```python
from build123d import *

# Parameters (mm, degrees)
F1_DEPTH = 3
F3_DEPTH = 3


with BuildPart() as f1:
    # F0 (on Front) → F1 (new body)
    with BuildSketch(Plane.XZ):
        with BuildLine():
            Line((-26.2521904707, -26.5712421387), (26.2521904707, -26.5712421387))
            ThreePointArc((26.2521904707, -26.5712421387), (29.7877243766, -25.1067760447), (31.2521904707, -21.5712421387))
            Line((31.2521904707, -21.5712421387), (31.2521904707, 21.5712421387))
            ThreePointArc((31.2521904707, 21.5712421387), (29.7877243766, 25.1067760447), (26.2521904707, 26.5712421387))
            Line((26.2521904707, 26.5712421387), (-26.2521904707, 26.5712421387))
            ThreePointArc((-26.2521904707, 26.5712421387), (-29.7877243766, 25.1067760447), (-31.2521904707, 21.5712421387))
            Line((-31.2521904707, 21.5712421387), (-31.2521904707, -21.5712421387))
            ThreePointArc((-31.2521904707, -21.5712421387), (-29.7877243766, -25.1067760447), (-26.2521904707, -26.5712421387))
        make_face()
        with BuildLine():
            Line((-24.1804867983, 6.5188668668), (-24.1804867983, 19.0295055509))
            Line((-24.1804867983, 19.0295055509), (-9.5692276955, 19.0295055509))
            Line((-9.5692276955, 19.0295055509), (-9.5692276955, 14.7253833711))
            Line((-9.5692276955, 14.7253833711), (-18.7460067018, 14.7253833711))
            ThreePointArc((-18.7460067018, 14.7253833711), (-19.0189579715, 14.6123232533), (-19.1320180893, 14.3393719836))
            Line((-19.1320180893, 14.3393719836), (-19.1320180893, 11.5628045595))
            ThreePointArc((-19.1320180893, 11.5628045595), (-19.052543922, 11.4032002875), (-18.8772828528, 11.3704401816))
            add(Edge.make_bspline(
                [(-18.8772828528, 11.3704401816), (-18.0907039553, 11.5942528357), (-16.428571119, 12.048986212), (-13.7637590064, 12.1663926481), (-10.7783023467, 11.2878918717), (-8.608008816, 8.883739189), (-7.8235892044, 7.195407339), (-7.479812433, 6.4214548917)],
                knots=[0.0187889452, 0.0187889452, 0.0187889452, 0.0187889452, 0.1928215696, 0.3859968189, 0.5892635727, 0.8004585236, 0.9781550685, 0.9781550685, 0.9781550685, 0.9781550685], degree=3))
            ThreePointArc((-7.479812433, 6.4214548917), (-7.1773938737, 6.1954394373), (-6.8268028651, 6.3355319618))
            add(Edge.make_bspline(
                [(-6.8268028651, 6.3355319618), (-6.3239368021, 6.9578108483), (-5.1657820011, 8.33523566), (-2.1396728387, 9.9326729538), (1.8950429815, 10.0853631714), (6.0194775368, 7.6605840045), (8.3949703412, 3.199174132), (8.7962173797, 0.4841619269), (8.9867115021, -0.8048042655)],
                knots=[0.0134429235, 0.0134429235, 0.0134429235, 0.0134429235, 0.1392843233, 0.2952512735, 0.4619051388, 0.6427907875, 0.8304130649, 1, 1, 1, 1], degree=3))
            Line((8.9867115021, -0.8048042655), (12.9019767046, -0.2800785005))
            add(Edge.make_bspline(
                [(12.9019767046, -0.2800785005), (13.0543244929, -1.4128068863), (13.328107964, -3.4484279333), (14.1004293769, -5.4535206804), (15.2062121625, -6.7542628508), (17.2121585921, -7.2105429933), (19.0659013385, -6.2089714944), (19.9198257488, -4.6565826928), (20.2026522486, -0.8100851133), (20.0692985967, 3.029626915), (20.2545182868, 5.7747033617), (18.5907316712, 8.3373482447), (16.4047076085, 8.7783260416), (14.8198998378, 8.6742253566), (13.28172228, 7.3709317022), (13.085235865, 6.1267789414), (12.9698067904, 5.5243223906)],
                knots=[0, 0, 0, 0, 0.0850530681, 0.1531982013, 0.2128134932, 0.2778382163, 0.3433024412, 0.4040377865, 0.4960108059, 0.5899390151, 0.6674603836, 0.7458264942, 0.8140016254, 0.8723646786, 0.9361011897, 1, 1, 1, 1], degree=3))
            Line((12.9698067904, 5.5243223906), (8.4308534861, 6.5188668668))
            Line((8.4308534861, 6.5188668668), (8.4308534861, 19.0295055509))
            Line((8.4308534861, 19.0295055509), (23.0421125889, 19.0295055509))
            Line((23.0421125889, 19.0295055509), (23.0421125889, 14.7253833711))
            Line((23.0421125889, 14.7253833711), (13.8653335825, 14.7253833711))
            ThreePointArc((13.8653335825, 14.7253833711), (13.5923823128, 14.6123232533), (13.4793221951, 14.3393719836))
            Line((13.4793221951, 14.3393719836), (13.4793221951, 11.5626012477))
            ThreePointArc((13.4793221951, 11.5626012477), (13.5587386682, 11.40304056), (13.7339183255, 11.370197343))
            add(Edge.make_bspline(
                [(13.7339183255, 11.370197343), (14.5206329081, 11.5934338311), (16.1829432155, 12.0472832886), (18.8464510581, 12.1747073507), (21.8375982381, 11.2543430537), (24.2004389296, 8.7818679608), (25.5755735256, 4.8713271716), (25.3064350862, -0.5737911857), (24.8312041176, -4.7094018545), (21.749976272, -9.0376680335), (16.9706732988, -10.4786564529), (12.5389209811, -9.3007692118), (10.8350653675, -7.5140693006), (10.3080651221, -6.5522620029)],
                knots=[0.006673314, 0.006673314, 0.006673314, 0.006673314, 0.0685294658, 0.1371846306, 0.2094263518, 0.2844857821, 0.3685608886, 0.4653028232, 0.5506041076, 0.6431140813, 0.7339975358, 0.8229147331, 0.8907000755, 0.8907000755, 0.8907000755, 0.8907000755], degree=3))
            ThreePointArc((10.3080651221, -6.5522620029), (9.8768736928, -6.3630255441), (9.583580391, -6.731421425))
            add(Edge.make_bspline(
                [(-8.4416717291, -13.5454395786), (-7.9438695099, -14.71578707), (-6.9579408758, -17.0337339557), (-4.2409263056, -19.6699254166), (0.459261844, -20.936928095), (5.9462638445, -19.1007566385), (8.4575100908, -14.8113966737), (9.4779663102, -10.267236628), (9.5666941787, -7.7613995922), (9.583580391, -6.731421425)],
                knots=[0, 0, 0, 0, 0.131573279, 0.2605891623, 0.4072468832, 0.5651074981, 0.7133867816, 0.8642572868, 0.9719474004, 0.9719474004, 0.9719474004, 0.9719474004], degree=3))
            Line((-8.4416717291, -13.5454395786), (-3.91946733, -12.3001933098))
            add(Edge.make_bspline(
                [(3.4391110044, -8.801032884), (3.4292294296, -9.8788771881), (3.3907020801, -12.0466383407), (2.98547267, -14.7224859441), (1.1638632401, -16.8474068921), (-1.2378962082, -16.8165054966), (-3.15517022, -15.3270751162), (-3.6508764536, -13.3639063953), (-3.91946733, -12.3001933098)],
                knots=[0.0310308646, 0.0310308646, 0.0310308646, 0.0310308646, 0.1949538702, 0.364973689, 0.5249423704, 0.6722147355, 0.8223945444, 1, 1, 1, 1], degree=3))
            ThreePointArc((3.4391110044, -8.801032884), (3.2178473715, -8.4483976929), (2.804982612, -8.5018005366))
            add(Edge.make_bspline(
                [(-7.6247713503, -5.0285945502), (-7.4951246028, -5.4581028515), (-7.1182427223, -6.5417591982), (-5.5143339169, -8.3435497571), (-1.8620178866, -10.0886878273), (1.4142697444, -9.5568731886), (2.461744348, -8.7898311991), (2.804982612, -8.5018005366)],
                knots=[0.0376498734, 0.0376498734, 0.0376498734, 0.0376498734, 0.1637941515, 0.3576495972, 0.6037857722, 0.8301707333, 0.9551635836, 0.9551635836, 0.9551635836, 0.9551635836], degree=3))
            ThreePointArc((-7.6247713503, -5.0285945502), (-7.954646037, -4.7561731868), (-8.3332477687, -4.9554002855))
            add(Edge.make_bspline(
                [(-23.6246287823, -0.8048042655), (-23.4238768593, -2.6360165944), (-23.0505161222, -6.0417263616), (-20.3186102891, -9.2347391659), (-15.6652683934, -10.4746071304), (-10.9657366753, -9.1109706503), (-8.8996831286, -5.9644979669), (-8.4359519706, -5.1438258987), (-8.3332477687, -4.9554002855)],
                knots=[0, 0, 0, 0, 0.1973470203, 0.3670282598, 0.5513187137, 0.7396844469, 0.9084969392, 0.9665234371, 0.9665234371, 0.9665234371, 0.9665234371], degree=3))
            Line((-23.6246287823, -0.8048042655), (-19.7093635798, -0.2800785005))
            add(Edge.make_bspline(
                [(-19.7093635798, -0.2800785005), (-19.5570157915, -1.4128068863), (-19.2832323204, -3.4484279333), (-18.5109109074, -5.4535206804), (-17.4051281218, -6.7542628508), (-15.3991816922, -7.2105429933), (-13.5454389459, -6.2089714944), (-12.6915145355, -4.6565826928), (-12.4086880358, -0.8100851133), (-12.5420416876, 3.029626915), (-12.3568219976, 5.7747033617), (-14.0206086131, 8.3373482447), (-16.2066326759, 8.7783260416), (-17.7914404465, 8.6742253566), (-19.3296180044, 7.3709317022), (-19.5261044193, 6.1267789414), (-19.641533494, 5.5243223906)],
                knots=[0, 0, 0, 0, 0.0850530681, 0.1531982013, 0.2128134932, 0.2778382163, 0.3433024412, 0.4040377865, 0.4960108059, 0.5899390151, 0.6674603836, 0.7458264942, 0.8140016254, 0.8723646786, 0.9361011897, 1, 1, 1, 1], degree=3))
            Line((-19.641533494, 5.5243223906), (-24.1804867983, 6.5188668668))
        make_face(mode=Mode.SUBTRACT)
    extrude(amount=F1_DEPTH)



with BuildPart() as f1b:
    # F0 (on Front) → F1, piece 2 (new body)
    with BuildSketch(Plane.XZ):
        with BuildLine():
            add(Edge.make_bspline(
                [(-3.4354478121, 1.6201604158), (-3.5268113996, 0.5204862984), (-3.661245232, -2.1514122715), (-2.8038980937, -5.0376153478), (-0.0082786462, -6.9479730958), (3.4625349906, -4.9889346896), (3.899180856, -0.526341138), (3.7411706941, 3.4063941992), (2.0399404478, 6.2494758513), (-0.4779286797, 6.4088353336), (-1.415072846, 5.9485227508), (-2.3566320655, 5.2360821356), (-3.2138401141, 3.6852138136), (-3.3662258173, 2.4533329967), (-3.4354478121, 1.6201604158)],
                knots=[0, 0, 0, 0, 0.1002894958, 0.1897756028, 0.2774641613, 0.3709145582, 0.478467765, 0.5828122225, 0.6726179006, 0.7498518805, 0.8019038103, 0.8568491044, 0.9240152544, 1, 1, 1, 1], degree=3))
        make_face()
    extrude(amount=F1_DEPTH)


with BuildPart() as f1_1:
    add(f1.part)

    add(f1b.part)  # F3 merges F1b
    # F2 (on face) → F3 (join)
    with BuildSketch(Plane.XZ):
        with BuildLine():
            Line((31.2521904707, -21.5712421387), (31.2521904707, 21.5712421387))
            ThreePointArc((31.2521904707, 21.5712421387), (29.7877243766, 25.1067760447), (26.2521904707, 26.5712421387))
            Line((26.2521904707, 26.5712421387), (-26.2521904707, 26.5712421387))
            ThreePointArc((-26.2521904707, 26.5712421387), (-29.7877243766, 25.1067760447), (-31.2521904707, 21.5712421387))
            Line((-31.2521904707, 21.5712421387), (-31.2521904707, -21.5712421387))
            ThreePointArc((-31.2521904707, -21.5712421387), (-29.7877243766, -25.1067760447), (-26.2521904707, -26.5712421387))
            Line((-26.2521904707, -26.5712421387), (26.2521904707, -26.5712421387))
            ThreePointArc((26.2521904707, -26.5712421387), (29.7877243766, -25.1067760447), (31.2521904707, -21.5712421387))
        make_face()
    extrude(amount=-F3_DEPTH)


solid = f1_1.part
```
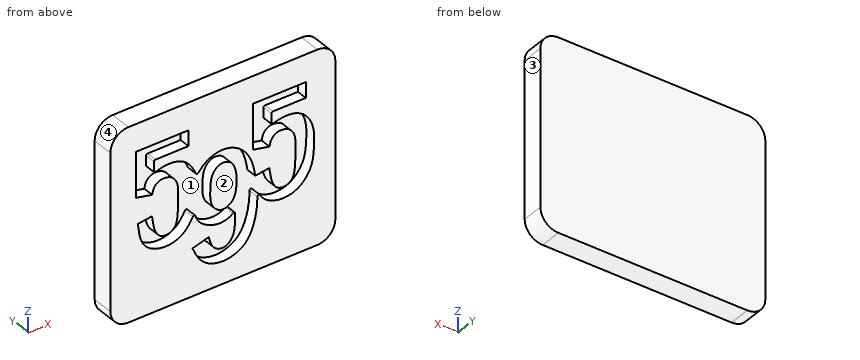
Could you check a few things on this model? Use its own coordinates, in mm. Face numbers are marked on the shaded views. Give positions to 0.01 mm unless a question says otherwise; leave off trailing zeros. Order: outer loops, then holes, each group sorted by start corner. A loop starts at its lowest first (then second) coordinate and runs counter-clockwise, first axis right, second up.
Q1. Suppose I cut it at B-B, the plane y = -1.75. Count the separate pieces of the cut face and the enclosed holes in it, and give its area (3 significant figures).
Q2. Suppose I cut it at A-A, the plane z = 13. Write out the boundary of the cut face in (x, y), and give its area (3 significant figures).
Q3. If I drill on line 1 along Z through (x, y) = (0, -1.75); line 2 along X through (y, z) = (-2, -6); line 3 along Z through (x, y) = (1.5, -1), over which ranges is the centre line in solid material (lowest first)?
Q4. We'd pull the mould along X, two halves only. Please class the marked faces 1, 2, 3 and 4: +X half, -X half, draft (parallel to the pull), parting line (faces both ways), or undercut.
Solution:
1. separate pieces: 2
1. enclosed holes: 1
1. area: 2,450 mm2
2. outline: (-31.25, -3) - (-24.18, -3) - (-24.18, 0) - (-19.13, 0) - (-19.13, -3) - (8.43, -3) - (8.43, 0) - (13.48, 0) - (13.48, -3) - (31.25, -3) - (31.25, 3) - (-31.25, 3) - close
2. area: 345 mm2
3. line 1: z = -26.57 to -20.42, -16.76 to -9.71, -6.32 to 6.32, 9.92 to 26.57
3. line 2: x = -31.25 to -22.57, -18 to -13.57, -8.95 to -7.27, -1.18 to 1.39, 14.61 to 19.04, 23.75 to 31.25
3. line 3: z = -26.57 to -20.31, -16.22 to -9.32, -5.94 to 6.02, 9.76 to 26.57
4. face 1: undercut
4. face 2: draft
4. face 3: +X half
4. face 4: -X half
